Job drawing, mm, ordinate dimensions from the low corner. One solid piece. Give positions to 0.01 mm unless a question says otherwise; leave off trailing zeros. Loops run counter-clockwise (first coordinate to the right, second up) from the corner with the lowest first, then second, coordinate; pieces in that order, holes last. Notation, with made-up numbers: (-37.75, -36) -> (-0.75, -36) arc R26 ccw to (-0.75, -14) -> close; hole circle Ø6 at (61.25, -6.75). An arc over 180 degrees is marked (long way). Answer as a JSON object with one key per item and string values. Group by question number.
Q1. Band-saw the part on C-C, the plane z = 68.5. Write the cut outline in (x, y).
Q2. Wall check: probe 1 along X at (y, z) = (0.55, 67.5); probe 2 along Z at (x, y) = (85.5, 0.45); probe 3 along X at (y, z) = (1, 6.5). Give the ranges that are in metal, low to high. Write a range as from..to.
Q3. Band-saw the part on B-B, the plane x = 6.5. Write the cut outline in (y, z), plus the area to 3 significant figures.
Q4. Drop a flat-ended pin along its axis: pin 1 (2.5 mm diameter, centred on x = 6.5, z = 68.5, fed in from -Y). Give the stop position or say it passes through.
Q5. Band-saw the part on A-A, the plane y = 0.65. Write the cut outline in (x, z).
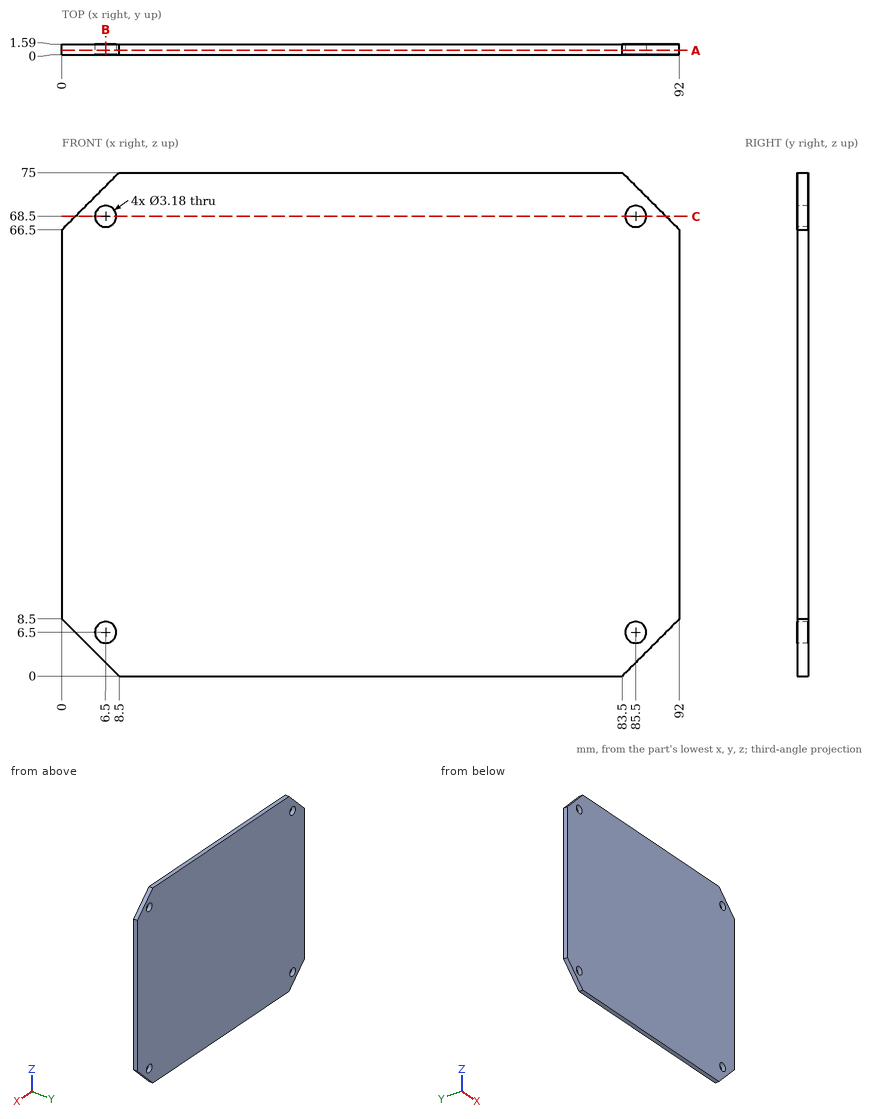
Worked answers:
{
 "1": {"outline": "(2, 0) -> (4.91, 0) -> (4.91, 1.59) -> (2, 1.59) -> close; (8.09, 0) -> (83.91, 0) -> (83.91, 1.59) -> (8.09, 1.59) -> close; (87.09, 0) -> (90, 0) -> (90, 1.59) -> (87.09, 1.59) -> close"},
 "2": {"probe 1": "1..5.26, 7.74..84.26, 86.74..91", "probe 2": "2..4.91, 8.09..66.91, 70.09..73", "probe 3": "2..4.91, 8.09..83.91, 87.09..90"},
 "3": {"outline": "(0, 2) -> (1.59, 2) -> (1.59, 4.91) -> (0, 4.91) -> close; (0, 8.09) -> (1.59, 8.09) -> (1.59, 66.91) -> (0, 66.91) -> close; (0, 70.09) -> (1.59, 70.09) -> (1.59, 73) -> (0, 73) -> close", "area": "103 mm2"},
 "4": {"pin 1": "through"},
 "5": {"outline": "(0, 8.5) -> (8.5, 0) -> (83.5, 0) -> (92, 8.5) -> (92, 66.5) -> (83.5, 75) -> (8.5, 75) -> (0, 66.5) -> close; hole circle Ø3.18 at (6.5, 6.5); hole circle Ø3.18 at (6.5, 68.5); hole circle Ø3.18 at (85.5, 6.5); hole circle Ø3.18 at (85.5, 68.5)"}
}
